Verification items for the finished model (mm, model axes). A direction names the side the tool comes from. Round coordinates to 2 decimals unless told otherwise and drop trailing zeros. Order: outer loops, then holes, each group sorted by start corner. A loop starts at its lowest first (then second) coordinate and runs counter-clockwise, first axis right, second up. Notation, with made-up numbers: (29, 5.25) -> (39, 5.25) arc R14 cw to (39, 18.25) -> close; hole circle Ø2 at (8.25, 7.5). An arc over 180 degrees is marked (long way). Return JSON: item names as keys, results as strings. Group by question number.
1) Depth check by flat-ended pin: pin 1 (8.5 mm diameter, centred on x = 2.75, z = -34, fed in from -Y); pin 2 (4 mm diameter, centred on y = 36.5, z = 25, fed in from +X); pin 3 (6 mm diameter, centred on x = 43, z = -29, fed in from +Y); pin 4 (20 mm diameter, centred on y = 60, z = -20, fed in from +X). Enter the tip coordinate at first touch or a pass-through.
2) Section check D-D on y = 66. Enter the section's corners in (x, z).
3) Section check C-C on z = -46. Enter the section's corners in (x, y).
4) Scan lines: L1, parallel to X at y = 48, z = -1.5; L2, parallel to Z at x = -10, y = 37; L3, parallel to Z at x = 2, y = 6. Record each from-to range of solid material in increasing order.
5) Section check B-B on x = 2.75. Enter the section's corners in (y, z), plus the area to 3 significant figures.
6) Section check A-A on z = 36. Enter the section's corners in (x, y).
7) Draft check along X on faces 6 (the flat face through (-7, 0, -13)), 7 (the flat face through (0, 45, -50)), 8 (the flat face through (-21, 34.5, -1)), 9 (the flat face through (-31.25, 39, 1)). Enter one of: pulls with the +X half, pulls with the -X half, needs draft (parallel to the pull), parting line crosses it, or undercut.
8) Tool access check on faces 1 (the cylindrical face through (7.11, 1.52, 14.83)), 2 (the flat face through (-26.25, 59, 1)), 3 (the cylindrical face through (46.04, 74.643, -23.252)), 4 (the flat face through (-11, 11, 12)), 5 (the flat face through (0, 39, 55)). Record the directions out of +Z, -Z, +X, -X, +Y, -Y that give a thin tool (end or side, any length) a straight path to the whole face; none if there is none.
```python
from build123d import *

# Parameters (mm, degrees)
SKETCH1_W                 = 62.5
SKETCH1_H                 = 110
BOSS_EXTRUDE1_DEPTH       = 80
SHELL1_T                  = -5
SHELL1_THICKNESS_2_FACE_W = 100
SHELL1_THICKNESS_2_FACE_H = 52.5
SHELL1_THICKNESS_2_DEPTH  = 6
SKETCH2_R                 = 15
SKETCH2_R_2               = 11
BOSS_EXTRUDE2_DEPTH       = 30
CUT_EXTRUDE2_REACH        = 117.461
BOSS_EXTRUDE3_START       = -52.5
BOSS_EXTRUDE3_DEPTH       = 10
CUT_EXTRUDE4_REACH        = 109.413
SKETCH6_R                 = 14.5
SKETCH6_3_R               = 16.002
SKETCH6_3_R_2             = 14.5
CUT_EXTRUDE5_DEPTH        = 8
SKETCH7_R                 = 4.7625
CUT_EXTRUDE6_DEPTH        = 108.413046228


with BuildPart() as part:
    # Sketch1 → Boss-Extrude1 (new body)
    with BuildSketch(Plane(origin=(0, 0, 0), x_dir=(1, 0, 0), z_dir=(0, 1, 0))):
        Rectangle(SKETCH1_W, SKETCH1_H)
    extrude(amount=BOSS_EXTRUDE1_DEPTH)

    # Shell1
    shell1_openings = [part.faces().sort_by_distance(p)[0] for p in [
        (0, 80, 0),
    ]]
    offset(amount=SHELL1_T, openings=shell1_openings, kind=Kind.INTERSECTION)

    # Shell1 thickness 2 face (on inner face of the shell) → Shell1 thickness 2 (add)
    with BuildSketch(Plane(origin=(0, 5, 0), x_dir=(0, 0, -1), z_dir=(0, -1, 0))):
        Rectangle(SHELL1_THICKNESS_2_FACE_W, SHELL1_THICKNESS_2_FACE_H)
    extrude(amount=-SHELL1_THICKNESS_2_DEPTH)

    # Sketch2 → Boss-Extrude2 (add)
    with BuildSketch(Plane(origin=(31.25, 0, 0), x_dir=(0, 0, -1), z_dir=(1, 0, 0))):
        with Locations(Location((20, 60, 0), (0, 0, 180))):
            Circle(SKETCH2_R)
        with Locations((20, 60)):
            Circle(SKETCH2_R_2, mode=Mode.SUBTRACT)
    extrude(amount=BOSS_EXTRUDE2_DEPTH)

    # Sketch2<3> → Cut-Extrude2 (cut, up to next)
    with BuildSketch(Plane(origin=(31.25, 0, 0), x_dir=(0, 0, -1), z_dir=(1, 0, 0)), mode=Mode.PRIVATE) as cut_extrude2_sk1:
        with BuildLine():
            ThreePointArc((31, 60), (27.778174593, 67.778174593), (20, 71))
            Line((20, 71), (20, 49))
            ThreePointArc((20, 49), (27.778174593, 52.221825407), (31, 60))
        make_face()
    cut_extrude2_tool1 = extrude(cut_extrude2_sk1.sketch, amount=-CUT_EXTRUDE2_REACH, mode=Mode.PRIVATE) & part.part
    # Sketch2<3> → Cut-Extrude2 (cut, up to next)
    with BuildSketch(Plane(origin=(31.25, 0, 0), x_dir=(0, 0, -1), z_dir=(1, 0, 0)), mode=Mode.PRIVATE) as cut_extrude2_sk2:
        with BuildLine():
            Line((20, 49), (20, 71))
            ThreePointArc((20, 71), (9, 60), (20, 49))
        make_face()
    cut_extrude2_tool2 = extrude(cut_extrude2_sk2.sketch, amount=-CUT_EXTRUDE2_REACH, mode=Mode.PRIVATE) & part.part
    # Sketch2<3> → Cut-Extrude2 (cut, up to next)
    with BuildSketch(Plane(origin=(31.25, 0, 0), x_dir=(0, 0, -1), z_dir=(1, 0, 0)), mode=Mode.PRIVATE) as cut_extrude2_sk3:
        with BuildLine():
            ThreePointArc((31, 60), (27.778174593, 67.778174593), (20, 71))
            Line((20, 71), (20, 49))
            ThreePointArc((20, 49), (27.778174593, 52.221825407), (31, 60))
        make_face()
    cut_extrude2_tool3 = extrude(cut_extrude2_sk3.sketch, amount=-CUT_EXTRUDE2_REACH, mode=Mode.PRIVATE) & part.part
    # Sketch2<3> → Cut-Extrude2 (cut, up to next)
    with BuildSketch(Plane(origin=(31.25, 0, 0), x_dir=(0, 0, -1), z_dir=(1, 0, 0)), mode=Mode.PRIVATE) as cut_extrude2_sk4:
        with BuildLine():
            Line((20, 49), (20, 71))
            ThreePointArc((20, 71), (9, 60), (20, 49))
        make_face()
    cut_extrude2_tool4 = extrude(cut_extrude2_sk4.sketch, amount=-CUT_EXTRUDE2_REACH, mode=Mode.PRIVATE) & part.part
    add(cut_extrude2_tool1.solids().sort_by_distance((31.25, 60, -24.668545))[0], mode=Mode.SUBTRACT)
    add(cut_extrude2_tool2.solids().sort_by_distance((31.25, 60, -15.331455))[0], mode=Mode.SUBTRACT)
    add(cut_extrude2_tool3.solids().sort_by_distance((31.25, 60, -24.668545))[0], mode=Mode.SUBTRACT)
    add(cut_extrude2_tool4.solids().sort_by_distance((31.25, 60, -15.331455))[0], mode=Mode.SUBTRACT)

    # 3DSketch1 → Boss-Extrude3 (add)
    with BuildSketch(Plane(origin=(26.25, 39.5, -50), x_dir=(0, -0.04993761694389221, 0.9987523388778448), z_dir=(1, 0, 0)).offset(BOSS_EXTRUDE3_START)):
        Polygon((0, 0), (0.249688085, 4.993761694), (100.124921973, 0), (99.875233888, -4.993761694), align=None)
    extrude(amount=BOSS_EXTRUDE3_DEPTH)

    # Sketch6 → Cut-Extrude4 (cut, up to next)
    with BuildSketch(Plane(origin=(0, 11, 0), x_dir=(1, 0, 0), z_dir=(0, 1, 0)), mode=Mode.PRIVATE) as cut_extrude4_sk1:
        with Locations(Location((2.75, -1, 0), (0, 0, 270))):
            Circle(SKETCH6_R)
    cut_extrude4_tool1 = extrude(cut_extrude4_sk1.sketch, amount=-CUT_EXTRUDE4_REACH, mode=Mode.PRIVATE) & part.part
    add(cut_extrude4_tool1.solids().sort_by_distance((2.75, 11, 1))[0], mode=Mode.SUBTRACT)

    # Sketch6<3> → Cut-Extrude5 (cut)
    with BuildSketch(Plane(origin=(0, 11, 0), x_dir=(1, 0, 0), z_dir=(0, 1, 0))):
        with Locations(Location((2.75, -1, 0), (0, 0, 270))):
            Circle(SKETCH6_3_R)
        with Locations(Location((2.75, -1, 0), (0, 0, 270))):
            Circle(SKETCH6_3_R_2, mode=Mode.SUBTRACT)
    extrude(amount=-CUT_EXTRUDE5_DEPTH, mode=Mode.SUBTRACT)

    # Sketch7 → Cut-Extrude6 (cut, through all)
    with BuildSketch(Plane(origin=(0, 11, 0), x_dir=(1, 0, 0), z_dir=(0, 1, 0))):
        with Locations(Location((2.75, -36, 0), (0, 0, 270))):
            Circle(SKETCH7_R)
        with Locations(Location((2.75, 34, 0), (0, 0, 270))):
            Circle(SKETCH7_R)
    extrude(amount=-CUT_EXTRUDE6_DEPTH, mode=Mode.SUBTRACT)


solid = part.part
```
Check result:
{
 "1": {"pin 1": "through", "pin 2": "x = 31.25", "pin 3": "y = 73.75", "pin 4": "x = -26.25"},
 "2": {"outline": "(-31.25, -55) -> (31.25, -55) -> (31.25, -33.75) -> (61.25, -33.75) -> (61.25, -29.22) -> (26.25, -29.22) -> (26.25, -50) -> (-26.25, -50) -> (-26.25, 50) -> (26.25, 50) -> (26.25, -10.78) -> (61.25, -10.78) -> (61.25, -6.25) -> (31.25, -6.25) -> (31.25, 55) -> (-31.25, 55) -> close"},
 "3": {"outline": "(-31.25, 0) -> (31.25, 0) -> (31.25, 80) -> (26.25, 80) -> (26.25, 11) -> (-26.25, 11) -> (-26.25, 34.5) -> (-16.25, 34.5) -> (-16.25, 39.5) -> (-26.25, 39.5) -> (-26.25, 80) -> (-31.25, 80) -> close"},
 "4": {"L1": "-31.25 to -26.25, 26.25 to 31.25", "L2": "-55 to -50, 50 to 55", "L3": "-55 to -38.7, -29.3 to -14.98, 16.98 to 31.3, 40.7 to 55"},
 "5": {"outline": "(0, -55) -> (80, -55) -> (80, -50) -> (11, -50) -> (11, -38.76) -> (0, -38.76) -> close; (0, -29.24) -> (11, -29.24) -> (11, -15) -> (3, -15) -> (3, -13.5) -> (0, -13.5) -> close; (0, 15.5) -> (3, 15.5) -> (3, 17) -> (11, 17) -> (11, 31.24) -> (0, 31.24) -> close; (0, 40.76) -> (11, 40.76) -> (11, 50) -> (80, 50) -> (80, 55) -> (0, 55) -> close", "area": "1,350 mm^2"},
 "6": {"outline": "(-31.25, 0) -> (-2.01, 0) -> (-2.01, 11) -> (-26.25, 11) -> (-26.25, 34.5) -> (-16.25, 34.5) -> (-16.25, 39.5) -> (-26.25, 39.5) -> (-26.25, 80) -> (-31.25, 80) -> close; (7.51, 0) -> (31.25, 0) -> (31.25, 80) -> (26.25, 80) -> (26.25, 11) -> (7.51, 11) -> close"},
 "7": {"face 6": "needs draft", "face 7": "undercut", "face 8": "undercut", "face 9": "pulls with the -X half"},
 "8": {"face 1": "+Y, -Y", "face 2": "+Y", "face 3": "+X", "face 4": "none", "face 5": "+Z, +X, -X, +Y, -Y"}
}
